Build history of the part. All positions in model axes, mm. A direction names the side the tool comes from. Round coordinates to 2 decimals unless told otherwise and drop trailing zeros. Loops run counter-clockwise (first coordinate to the right, second up) from the corner with the lowest first, then second, coordinate; pieces in that order, holes last. Notation, with made-up numbers: (23.25, 77.25) - (53.25, 77.25) arc R19 cw to (53.25, 94.25) - close; hole circle Ø6 at (86, 72.5). An arc over 180 degrees is marked (long way). Use a Markdown table: item, result.
from build123d import *

# Parameters (mm, degrees)
SKETCH2_W           = 254
SKETCH2_H           = 41
BOSS_EXTRUDE1_DEPTH = 40
SKETCH3_W           = 44.69
SKETCH3_H           = 40
BOSS_EXTRUDE6_DEPTH = 55.6
SKETCH7_W           = 100
SKETCH7_H           = 40
BOSS_EXTRUDE7_DEPTH = 55.6
SKETCH8_W           = 41
SKETCH8_H           = 40
BOSS_EXTRUDE8_DEPTH = 150
SKETCH9_W           = 40
SKETCH9_H           = 45
BOSS_EXTRUDE9_DEPTH = 55.6


with BuildPart() as part:
    # Sketch2 → Boss-Extrude1 (new body)
    with BuildSketch(Plane.XY):
        with Locations((-241.745614035, -30.596491228)):
            Rectangle(SKETCH2_W, SKETCH2_H)
        with Locations((12.254385965, -30.596491228)):
            Rectangle(SKETCH2_W, SKETCH2_H)
    extrude(amount=BOSS_EXTRUDE1_DEPTH)

    # Sketch3 → Boss-Extrude6 (add)
    with BuildSketch(Plane(origin=(0, 0, 0), x_dir=(-1, 0, 0), z_dir=(0, 0, -1))):
        with Locations((373.090614035, -31.096491228)):
            Rectangle(SKETCH3_W, SKETCH3_H)
    extrude(amount=BOSS_EXTRUDE6_DEPTH)

    # Sketch7 → Boss-Extrude7 (add)
    with BuildSketch(Plane(origin=(0, 0, 0), x_dir=(-1, 0, 0), z_dir=(0, 0, -1))):
        with Locations((-134.464385965, -31.096491228)):
            Rectangle(SKETCH7_W, SKETCH7_H)
    extrude(amount=BOSS_EXTRUDE7_DEPTH)

    # Sketch8 → Boss-Extrude8 (add)
    with BuildSketch(Plane.XZ.offset(51.096491228)):
        with Locations((118.754385965, 20)):
            Rectangle(SKETCH8_W, SKETCH8_H)
        with Locations((-348.245614035, 20)):
            Rectangle(SKETCH8_W, SKETCH8_H)
    extrude(amount=BOSS_EXTRUDE8_DEPTH)

    # Sketch9 → Boss-Extrude9 (add)
    with BuildSketch(Plane(origin=(0, 0, 0), x_dir=(-1, 0, 0), z_dir=(0, 0, -1))):
        with Locations((-119.154385965, -89.642057698)):
            Rectangle(SKETCH9_W, SKETCH9_H)
        with Locations((348.645614035, -89.642057698)):
            Rectangle(SKETCH9_W, SKETCH9_H)
    extrude(amount=BOSS_EXTRUDE9_DEPTH)


solid = part.part
Q1. Cut at D-D, the plane z = 29. List the corners of the cut face in (x, y).
Results found:
| item | result |
|---|---|
| outline | (-368.75, -201.1) - (-327.75, -201.1) - (-327.75, -51.1) - (98.25, -51.1) - (98.25, -201.1) - (139.25, -201.1) - (139.25, -10.1) - (-368.75, -10.1) - close |
Q2. Probe line 1 (X direction, y = -164.5, z = 8); line 2 (Y direction, x = -6, z = 15.5); line 3 (X direction, y = -19, z = 6). List the from-to ranges inside material, lowest first.
Results found:
| item | result |
|---|---|
| line 1 | x = -368.75 to -327.75, 98.25 to 139.25 |
| line 2 | y = -51.1 to -10.1 |
| line 3 | x = -368.75 to 139.25 |
Q3. Cut at A-A, the plane z = -27. List the corners of the cut face in (x, y), plus the area to 3 significant figures.
Results found:
| item | result |
|---|---|
| outline | (-395.44, -51.1) - (-350.75, -51.1) - (-350.75, -11.1) - (-395.44, -11.1) - close; (-368.65, -112.14) - (-328.65, -112.14) - (-328.65, -67.14) - (-368.65, -67.14) - close; (84.46, -51.1) - (184.46, -51.1) - (184.46, -11.1) - (84.46, -11.1) - close; (99.15, -112.14) - (139.15, -112.14) - (139.15, -67.14) - (99.15, -67.14) - close |
| area | 9,390 mm2 |
Q4. Cut at C-C, the plane y = -33. List the corners of the cut face in (x, z).
Results found:
| item | result |
|---|---|
| outline | (-395.44, -55.6) - (-350.75, -55.6) - (-350.75, 0) - (84.46, 0) - (84.46, -55.6) - (184.46, -55.6) - (184.46, 0) - (139.25, 0) - (139.25, 40) - (-368.75, 40) - (-368.75, 0) - (-395.44, 0) - close |
Q5. Which spindle directions (+Z, -Z, +X, -X, +Y, -Y) get a long thin tool onto all of the face, cutting with end or side? Do faces 1 (the face through (119, -67.142, -27)), 2 (the face through (135, -11.096, -27)). Say none if no direction does.
Results found:
| item | result |
|---|---|
| face 1 | -Z, +X, -X |
| face 2 | -Z, +X, -X, +Y |
Q6. Drop flat-ended pins along their axis: pin 1 (5 mm diameter, centred on x = -104.5, y = -30, fed in from -Z); pin 2 (4 mm diameter, centred on x = -226.5, z = 9.5, fed in from -Y); pin 3 (10 mm diameter, centred on x = -278, y = -56.5, fed in from +Z) (1 decimal); pin 4 (20 mm diameter, centred on y = -119, z = 27.5, fed in from -X). Give the stop position or say it passes through.
Results found:
| item | result |
|---|---|
| pin 1 | stops at z = 0 |
| pin 2 | stops at y = -51.1 |
| pin 3 | passes through |
| pin 4 | stops at x = -368.75 |
Q7. Cut at B-B, the plane y = -79. List the corners of the cut face in (x, z), plus the area to 3 significant figures.
Results found:
| item | result |
|---|---|
| outline | (-368.75, 0) - (-368.65, 0) - (-368.65, -55.6) - (-328.65, -55.6) - (-328.65, 0) - (-327.75, 0) - (-327.75, 40) - (-368.75, 40) - close; (98.25, 0) - (99.15, 0) - (99.15, -55.6) - (139.15, -55.6) - (139.15, 0) - (139.25, 0) - (139.25, 40) - (98.25, 40) - close |
| area | 7,730 mm2 |
